from build123d import *

# Parameters (mm, degrees)
BOSS_EXTRUDE1_DEPTH              = 10
SKETCH2_W                        = 10
SKETCH2_H                        = 7
CUT_EXTRUDE2_DEPTH               = 71
CUT_EXTRUDE3_DEPTH               = 71
F_5_0_19685_DIAMETER_HOLE1_D     = 4.99999
F_5_0_19685_DIAMETER_HOLE1_DEPTH = 10
F_5_0_19685_DIAMETER_HOLE1_TIP   = 1.502148543
CUT_EXTRUDE4_REACH               = 43.061
CUT_EXTRUDE4_END_RADIUS          = 2.499995
SKETCH8_R                        = 2.25
CHAMFER1_SIZE                    = 0.5


with BuildPart() as part:
    # Sketch1 → Boss-Extrude1 (new body)
    with BuildSketch(Plane(origin=(0, 0, 0), x_dir=(1, 0, 0), z_dir=(0, 1, 0))):
        Polygon((-10, 7), (-10, 19), (5, 19), (5, 7), (25, 7), (25, -7), (-25, -7), (-25, 7), align=None)
    extrude(amount=BOSS_EXTRUDE1_DEPTH)

    # Sketch2 → Cut-Extrude2 (cut)
    with BuildSketch(Plane.ZY.offset(25)):
        with Locations((0, 6.5)):
            Rectangle(SKETCH2_W, SKETCH2_H)
    extrude(amount=-CUT_EXTRUDE2_DEPTH, mode=Mode.SUBTRACT)

    # Sketch4 → Cut-Extrude3 (cut)
    with BuildSketch(Plane(origin=(0, 0, 0), x_dir=(1, 0, 0), z_dir=(0, 1, 0))):
        with BuildLine():
            Line((-16, 3), (16, 3))
            ThreePointArc((16, 3), (19, 0), (16, -3))
            Line((16, -3), (-16, -3))
            ThreePointArc((-16, -3), (-19, 0), (-16, 3))
        make_face()
    extrude(amount=CUT_EXTRUDE3_DEPTH, mode=Mode.SUBTRACT)

    # #5 (0.19685) Diameter Hole1
    with Locations(Plane(origin=(0, 0, -19), x_dir=(-1, 0, 0), z_dir=(0, 0, -1))):
        with Locations((0, 5)):
            Hole(F_5_0_19685_DIAMETER_HOLE1_D / 2, depth=F_5_0_19685_DIAMETER_HOLE1_DEPTH)
            with Locations((0, 0, -(F_5_0_19685_DIAMETER_HOLE1_DEPTH + F_5_0_19685_DIAMETER_HOLE1_TIP / 2))):  # 118° drill point
                Cone(0, F_5_0_19685_DIAMETER_HOLE1_D / 2, F_5_0_19685_DIAMETER_HOLE1_TIP, mode=Mode.SUBTRACT)

    # Cut-Extrude4: up to this cylinder (the profile starts outside it)
    cut_extrude4_end = Plane(origin=(0, 5, -13), z_dir=(0, 0, -1)) * Cylinder(CUT_EXTRUDE4_END_RADIUS, 92.12199, mode=Mode.PRIVATE)
    # Sketch8 → Cut-Extrude4 (cut, up to the surface)
    with BuildSketch(Plane.ZY.offset(10), mode=Mode.PRIVATE) as cut_extrude4_sk1:
        with Locations((-13, 5)):
            Circle(SKETCH8_R)
    cut_extrude4_tool1 = extrude(cut_extrude4_sk1.sketch, amount=-CUT_EXTRUDE4_REACH, mode=Mode.PRIVATE) - cut_extrude4_end
    add(cut_extrude4_tool1.solids().sort_by_distance((-10, 5, -13))[0], mode=Mode.SUBTRACT)

    # Chamfer1
    chamfer1_edges = [part.edges().sort_by_distance(p)[0] for p in [
        (0, 3, -3),
        (19, 3, 0),
        (0, 3, 3),
        (-19, 3, 0),
        (-19, 0, 0),
        (0, 0, 3),
        (19, 0, 0),
        (0, 0, -3),
        (-2.499995, 5, -19),
        (-10, 5, -15.25),
    ]]
    chamfer(chamfer1_edges, length=CHAMFER1_SIZE)


solid = part.part
Input: part model. Units: mm. Frame: model coordinates. A direction names the side the tool comes from. Coordinates: 2 decimals unless noted, no trailing zeros. Order: outer loops, then holes, each group sorted by start corner. A loop starts at its lowest first (then second) coordinate and runs counter-clockwise, first axis right, second up. Notation, with made-up numbers: M -33.75,-40 L 18.25,-40 A14 ccw 18.25,-22 Z; hole C -5,31 d9. An arc over 180 degrees is marked long. Write item = value, one per line. Start each with the question number.
(1) Section B-B on x = -11.5. Output: boundary loops of the cut face in (y, z), and give its area (3 significant figures).
(2) Reachability of faces 5 (the flat face through (15, 5, -7)), 6 (the conical face through (-19.135, 0.365, 0.069)), 7 (the cylindrical face through (2.31, 4.04, -13.68)), 8 (the conical face through (19.14, 2.64, -0.07)) from +Z, -Z, +X, -X, +Y, -Y: full face, straight path, thin tool, end or side. Return the list, or none.
(3) Section D-D on z = 0. Output: boundary loops of the cut face in (x, y).
(4) Section C-C on x = -5.5. Output: boundary loops of the cut face in (y, z), and give its area (3 significant figures).
(5) Section A-A on y = 9.5. Output: boundary loops of the cut face in (x, z), and give its area (3 significant figures).
(6) Line query: line 1 along Z through (x, y) = (-3.25, 5); line 2 along Y through (x, z) = (-7.25, -13); line 3 along Z through (x, y) = (21, 5). Output: solid intervals per line, ascending. Write a range as [from, to].
(7) Pull-direction query (X, two-part tool) for faces 1 (the conical face through (-19.14, 2.64, 0.07)), 2 (the flat face through (0, 1, 3)), 3 (the flat face through (-25, 2.7, 0.1)), 4 (the cylindrical face through (-5.353, 2.804, -13.488)); classes: released by +X, released by -X, zero draft, split by the parting line, or undercut.
(8) First-contact query: P1, Ø3, axis at y = 4, z = -12.5, coming from the -X side; P2, Ø4, axis at x = -19, z = -10, coming from the +Y side; P3, Ø5, axis at y = 3.5, z = -13, coming from the +X side; P4, Ø5, axis at y = 5, z = -13, coming from the -X side. Flat tips, straight axial feed; report the tip coordinate or a pass-through.
Result set:
q1.outline = M 0,-7 L 10,-7 L 10,-5 L 3,-5 L 3,-3.5 L 2.5,-3 L 0.5,-3 L 0,-3.5 Z; M 0,3.5 L 0.5,3 L 2.5,3 L 3,3.5 L 3,5 L 10,5 L 10,7 L 0,7 Z
q1.area = 51.5 mm²
q2.face_5 = -Z, +X, +Y, -Y
q2.face_6 = -Y
q2.face_7 = -Z
q2.face_8 = +Y
q3.outline = M -25,0 L -19.5,0 L -19,0.5 L -19,2.5 L -19.5,3 L -25,3 Z; M 19,0.5 L 19.5,0 L 25,0 L 25,3 L 19.5,3 L 19,2.5 Z
q4.outline = M 0,-19 L 10,-19 L 10,-5 L 3,-5 L 3,-3.5 L 2.5,-3 L 0.5,-3 L 0,-3.5 Z; M 0,3.5 L 0.5,3 L 2.5,3 L 3,3.5 L 3,5 L 10,5 L 10,7 L 0,7 Z; hole C 5,-13 d4.5
q4.area = 156 mm²
q5.outline = M -25,-7 L -10,-7 L -10,-19 L 5,-19 L 5,-7 L 25,-7 L 25,-5 L -25,-5 Z; M -25,5 L 25,5 L 25,7 L -25,7 Z
q5.area = 380 mm²
q6.line_1 = [-19, -15.25], [-10.75, -5], [5, 7]
q6.line_2 = [0, 2.75], [7.25, 10]
q6.line_3 = [-7, -5], [5, 7]
q7.face_1 = undercut
q7.face_2 = undercut
q7.face_3 = released by -X
q7.face_4 = zero draft
q8.P1 = -9.87
q8.P2 = through
q8.P3 = 5
q8.P4 = -9.75
